Could you check a few things on this model? Use its own coordinates, in mm. Give positions to 0.01 mm unless a question says otherwise; leave off trailing zeros. Loops run counter-clockwise (first coordinate to the right, second up) from the corner with the lowest first, then second, coordinate; pieces in that order, holes last. Notation, with made-up numbers: (-19, -2) - (40, -2) arc R29 cw to (40, 31) - close; hole circle Ø10 at (5, 43). An arc over 180 degrees is marked (long way). One line per item, written item: value. Start each with the question number.
Q1. I want a section at A-A (z = -1.75). Please give me the cut outline in (x, y).
Q2. I want a section at C-C (z = -8.25). Please give me the cut outline in (x, y), then the cut area to 3 significant figures.
Q3. I want a section at B-B (y = -2.65). Please give me the cut outline in (x, z).
Q4. If we mould it in two halves opening along Z, with no side actions, what happens to faces 1 (the face through (37.242, -1.932, -4.71)), 2 (the face through (22.92, -1.93, -6.58)), 3 (the face through (0, -2, -9.712)), 4 (the face through (0, -2, 0))? For each: released by +Z, released by -Z, zero draft, split by the parting line, or undercut.
Q5. If I drill on line 1 (X direction, y = -1.1, z = -4.5); line 2 (X direction, y = -3.05, z = -5); line 3 (Z direction, x = 19, y = -0.95), over which ranges is the centre line in solid material (lowest first)? Write a range as from..to.
```python
from build123d import *

# Parameters (mm, degrees)
F0_W     = 120.43124
F0_H     = 9.712197
F1_DEPTH = 3.81
F2_R     = 4.385573
F3_DEPTH = 38.1
F4_R     = 0.508


with BuildPart() as f1:
    # F0 (on Front) → F1 (new body)
    with BuildSketch(Plane.XZ):
        with Locations((0.832474, -4.856098)):
            Rectangle(F0_W, F0_H)
    extrude(amount=F1_DEPTH)

    # F2 (on face) → F3 (cut)
    with BuildSketch(Plane.XZ.offset(3.81)):
        with Locations((18.869411, -4.902347)):
            Circle(F2_R)
        with Locations((30.709038, -4.902347)):
            Circle(F2_R)
        with Locations((41.6237, -4.902347)):
            Circle(F2_R)
        with Locations((54.203305, -4.902347)):
            Circle(F2_R)
    extrude(amount=-F3_DEPTH, mode=Mode.SUBTRACT)

    # F4
    f4_edges = [f1.edges().sort_by_distance(p)[0] for p in [
        (-59.383146, -3.81, -4.856098),
        (-59.383146, 0, -4.856098),
        (61.048094, 0, -4.856098),
        (61.048094, -3.81, -4.856098),
    ]]
    fillet(f4_edges, radius=F4_R)


solid = f1.part
```
Worked answers:
1. outline: (-59.38, -3.3) arc R0.51 ccw to (-58.88, -3.81) - (15.82, -3.81) - (15.82, 0) - (-58.88, 0) arc R0.51 ccw to (-59.38, -0.51) - close; (21.92, -3.81) - (27.66, -3.81) - (27.66, 0) - (21.92, 0) - close; (33.76, -3.81) - (38.57, -3.81) - (38.57, 0) - (33.76, 0) - close; (44.67, -3.81) - (51.15, -3.81) - (51.15, 0) - (44.67, 0) - close; (57.25, -3.81) - (60.54, -3.81) arc R0.51 ccw to (61.05, -3.3) - (61.05, -0.51) arc R0.51 ccw to (60.54, 0) - (57.25, 0) - close
2. outline: (-59.38, -3.3) arc R0.51 ccw to (-58.88, -3.81) - (16.04, -3.81) - (16.04, 0) - (-58.88, 0) arc R0.51 ccw to (-59.38, -0.51) - close; (21.7, -3.81) - (27.88, -3.81) - (27.88, 0) - (21.7, 0) - close; (33.54, -3.81) - (38.79, -3.81) - (38.79, 0) - (33.54, 0) - close; (44.46, -3.81) - (51.37, -3.81) - (51.37, 0) - (44.46, 0) - close; (57.04, -3.81) - (60.54, -3.81) arc R0.51 ccw to (61.05, -3.3) - (61.05, -0.51) arc R0.51 ccw to (60.54, 0) - (57.04, 0) - close
2. area: 372 mm²
3. outline: (-59.38, -9.71) - (61.05, -9.71) - (61.05, 0) - (-59.38, 0) - close; hole circle Ø8.77 at (18.87, -4.9); hole circle Ø8.77 at (30.71, -4.9); hole circle Ø8.77 at (41.62, -4.9); hole circle Ø8.77 at (54.2, -4.9)
4. face 1: undercut
4. face 2: undercut
4. face 3: released by -Z
4. face 4: released by +Z
5. line 1: x = -59.38..14.5, 23.24..26.34, 35.08..37.26, 45.99..49.84, 58.57..61.05
5. line 2: x = -59.38..14.48, 23.25..26.32, 35.09..37.24, 46.01..49.82, 58.59..61.05
5. line 3: z = -9.71..-9.29, -0.52..0
